CAD build for the part. Positions are in the model's coordinates, mm. Face numbers are marked on the shaded views. A direction names the side the tool comes from. Coordinates: 2 decimals unless noted, no trailing zeros. Order: outer loops, then holes, each group sorted by start corner. A loop starts at its lowest first (then second) coordinate and runs counter-clockwise, first axis right, second up. Notation, with made-up numbers: (85, -13) - (138, -13) arc R18 cw to (138, -2) - close; hole circle Ø4 at (23, 7). An arc over 180 degrees is marked (long way). Use one line per item in the form item = value.
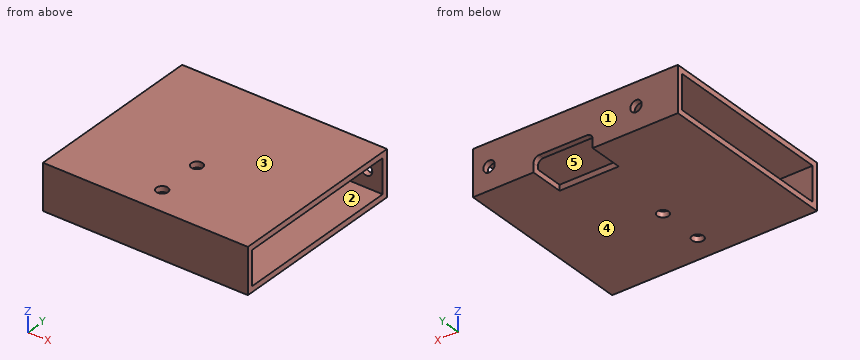
Autodesk Inventor part; units mm, degrees
ref_plane "YZ Plane" through (0, 0, 0) normal (1, 0, 0) x (0, 1, 0)
ref_plane "XZ Plane" through (0, 0, 0) normal (0, 1, 0) x (-1, 0, 0)
ref_plane "XY Plane" through (0, 0, 0) normal (0, 0, 1) x (1, 0, 0)
sketch "Sketch1" plane through (0, 0, 0) normal (1, 0, 0) x (0, 1, 0)
  line L0 (0, 0) -> (-101.6, 0)
  line L1 (-101.6, 0) -> (-101.6, -25.4)
  line L2 (-101.6, -25.4) -> (0, -25.4)
  line L3 (0, -25.4) -> (0, 0)
  line L4 (-3.175, -22.225) -> (-98.425, -22.225)
  line L5 (-98.425, -22.225) -> (-98.425, -3.175)
  line L6 (-98.425, -3.175) -> (-3.175, -3.175)
  line L7 (-3.175, -3.175) -> (-3.175, -22.225)
  dimension "d0" = 101.6
  dimension "d1" = 25.4
  dimension "d2" = 3.175
extrude "Extrusion1" add sketch "Sketch1" along normal blind 114.3
sketch "Sketch2" plane through (0, 0, 0) normal (0, 1, 0) x (1, 0, 0)
  line L0 (0, 25.4) -> (0, 0)
  line L1 (0, 0) -> (114.3, 0)
  line L2 (114.3, 25.4) -> (114.3, 0)
  line L3 (0, 25.4) -> (114.3, 25.4)
  circle A0 centre (64.3357, 49.9643) radius 6.35
  circle A1 centre (64.3357, 49.9643) radius 28.3845
extrude "Extrusion2" cut sketch "Sketch2" against normal blind 19.05 contours A1 L3 | L3 A1
sketch "Sketch3" plane through (0, 0, 0) normal (0, 1, 0) x (1, 0, 0)
  circle A0 centre (23.3357, 12.7) radius 3.175
  circle A1 centre (105.3357, 12.7) radius 3.175
  point P0 (0, 0)
extrude "Extrusion3" cut sketch "Sketch3" against normal blind 12.7
sketch "Sketch4" plane through (0, -101.6, 0) normal (0, 0, 1) x (1, 0, 0)
  point P0 (0, 101.6)
  point P1 (55.5752, 14.3002)
  point P2 (55.5752, 39.7002)
hole "Hole1" at (55.5752, -87.2998, 0) at (55.5752, -61.8998, 0) direction (0, 0, -1) diameter 6.35 end through all
sketch "Sketch5" plane through (0, 0, 0) normal (0, 1, 0) x (1, 0, 0)
  circle A0 centre (23.3357, 12.7) radius 3.175
  circle A1 centre (105.3357, 12.7) radius 3.175
  arc A2 (50.1134, 25.4) -> (78.5579, 25.4) centre (64.3357, 49.9643) ccw
  line L0 (0, 25.4) -> (50.1134, 25.4)
  line L1 (0, 25.4) -> (0, 0)
  line L2 (0, 0) -> (114.3, 0)
  line L3 (114.3, 25.4) -> (114.3, 0)
  line L4 (78.5579, 25.4) -> (114.3, 25.4)
  line L5 (0, 25.4) -> (50.1134, 25.4)
  line L6 (47.5287, 25.4) -> (80.556, 25.4)
  line L7 (80.556, 25.4) -> (80.556, 17.4223)
  line L8 (80.556, 17.4223) -> (47.5287, 17.4223)
  line L9 (47.5287, 17.4223) -> (47.5287, 25.4)
extrude "Extrusion4" cut sketch "Sketch5" against normal blind 19.05 contours L6 A2 | A2 L4 L7 L8 L9 L0
fillet "Fillet1" radius 3.175 1 edges at (47.5287, -1.5875, -17.4223)
fillet "Fillet2" radius 3.175 1 edges at (80.556, -1.5875, -17.4223)
properties part number "Front Fender BoxBeam"
Item 1: Two-plate mould, pull along Z, no slides. Class the marked faces 3, 4 and 5: +Z half, -Z half, draft (parallel to the pull), parting line (faces both ways), or undercut.
Derived:
face_3 = +Z half
face_4 = -Z half
face_5 = undercut
Item 2: 3-axis set-ups, long thin cutter, end or side, ignore diameter. For the marked faces 1 and 2: which of +Z, -Z, +X, -X, +Y, -Y reach the whole face in a straight line?
Derived:
face_1 = +Z, -Z, +X, -X, +Y
face_2 = +X, -X
Item 3: Cut at D-D, the plane y = -10. Write the cut outline in (x, z) (3 decimals).
Derived:
outline = (0, -25.4) - (47.529, -25.4) - (47.529, -22.225) - (0, -22.225) - close; (0, -3.175) - (114.3, -3.175) - (114.3, 0) - (0, 0) - close; (80.556, -25.4) - (114.3, -25.4) - (114.3, -22.225) - (80.556, -22.225) - close
Item 4: Cut at C-C, the plane x = 89. Write the cut outline in (y, z) (3 decimals).
Derived:
outline = (-101.6, -25.4) - (0, -25.4) - (0, 0) - (-101.6, 0) - close; hole (-98.425, -22.225) - (-3.175, -22.225) - (-3.175, -3.175) - (-98.425, -3.175) - close
Item 5: Cut at A-A, the plane y = -76.5. Write the cut outline in (x, z) (3 decimals).
Derived:
outline = (0, -25.4) - (114.3, -25.4) - (114.3, -22.225) - (0, -22.225) - close; (0, -3.175) - (114.3, -3.175) - (114.3, 0) - (0, 0) - close
Item 6: Cut at B-B, the plane z = -12.7. Write the cut outline in (x, y) (3 decimals), plus the area to 3 significant figures.
Derived:
outline = (0, -101.6) - (114.3, -101.6) - (114.3, -98.425) - (0, -98.425) - close; (0, -3.175) - (20.161, -3.175) - (20.161, 0) - (0, 0) - close; (26.511, -3.175) - (102.161, -3.175) - (102.161, 0) - (26.511, 0) - close; (108.511, -3.175) - (114.3, -3.175) - (114.3, 0) - (108.511, 0) - close
area = 685 mm²
Item 7: Drop flat-ended pins along their axis: pin 1 (1.6 mm diameter, centred on x = 68.5, z = -24.5, fed in from +Y); pin 2 (1.6 mm diameter, centred on x = 62, y = -1.5, fed in from -Z); pin 3 (5.5 mm diameter, centred on x = 105.34, z = -12.7, fed in from +Y) (3 decimals). Give the stop position or say it passes through.
Derived:
pin_1 = -19.05
pin_2 = -17.42
pin_3 = -98.425
Item 8: Drill centre lines: line 1 (X direction, y = -1.5, z = -12.7); line 2 (Y direction, x = 69, z = -11.25) (3 decimals); line 3 (Z direction, x = 20, y = -20.5) (3 decimals). Where is each one in solid material? Low to high. Write a range as [from, to].
Derived:
line_1 = [0, 20.16], [26.51, 102.16], [108.51, 114.3]
line_2 = [-101.6, -98.425], [-3.175, 0]
line_3 = [-25.4, -22.225], [-3.175, 0]
